Design review of the part built by this model. Coordinates are the model's own, in mm. A direction names the side the tool comes from. Coordinates: 2 decimals unless noted, no trailing zeros. Loops run counter-clockwise (first coordinate to the right, second up) from the corner with the lowest first, then second, coordinate; pieces in that order, holes last.
from build123d import *

# Parameters (mm, degrees)
SKETCH1_W           = 18.669
SKETCH1_H           = 50.8
BOSS_EXTRUDE1_DEPTH = 44.069
SKETCH2_W           = 44.069
SKETCH2_H           = 4.7625
CUT_EXTRUDE1_DEPTH  = 70.794328724
SKETCH3_W           = 44.069
SKETCH3_H           = 14.29004
CUT_EXTRUDE2_DEPTH  = 4.7625
SKETCH5_W           = 44.069
SKETCH5_H           = 14.29004
CUT_EXTRUDE3_DEPTH  = 4.7625
SKETCH4_W           = 18.669
SKETCH4_H           = 14.29004
CUT_EXTRUDE4_DEPTH  = 4.7625
SKETCH6_W           = 18.669
SKETCH6_H           = 14.29004
CUT_EXTRUDE5_DEPTH  = 4.7625
FILLET1_R           = 4.50088
FILLET2_R           = 2.49936
SKETCH7_R           = 2.5527
SKETCH7_R_2         = 2.54
CUT_EXTRUDE6_DEPTH  = 70.794328724
SKETCH8_R           = 2.0193
CUT_EXTRUDE7_DEPTH  = 69.673921566


with BuildPart() as part:
    # Sketch1 → Boss-Extrude1 (new body)
    with BuildSketch(Plane.XY):
        with Locations((9.3345, 25.4)):
            Rectangle(SKETCH1_W, SKETCH1_H)
    extrude(amount=BOSS_EXTRUDE1_DEPTH)

    # Sketch2 → Cut-Extrude1 (cut, through all)
    with BuildSketch(Plane(origin=(18.669, 0, 0), x_dir=(0, 0, -1), z_dir=(1, 0, 0))):
        with Locations((-22.0345, 2.38125)):
            Rectangle(SKETCH2_W, SKETCH2_H)
    extrude(amount=-CUT_EXTRUDE1_DEPTH, mode=Mode.SUBTRACT)

    # Sketch3 → Cut-Extrude2 (cut)
    with BuildSketch(Plane(origin=(18.669, 0, 0), x_dir=(0, 0, -1), z_dir=(1, 0, 0))):
        with Locations((-22.0345, 11.90752)):
            Rectangle(SKETCH3_W, SKETCH3_H)
    extrude(amount=-CUT_EXTRUDE2_DEPTH, mode=Mode.SUBTRACT)

    # Sketch5 → Cut-Extrude3 (cut)
    with BuildSketch(Plane.ZY):
        with Locations((22.0345, 11.90752)):
            Rectangle(SKETCH5_W, SKETCH5_H)
    extrude(amount=-CUT_EXTRUDE3_DEPTH, mode=Mode.SUBTRACT)

    # Sketch4 → Cut-Extrude4 (cut)
    with BuildSketch(Plane.XY.offset(44.069)):
        with Locations((9.3345, 11.90752)):
            Rectangle(SKETCH4_W, SKETCH4_H)
    extrude(amount=-CUT_EXTRUDE4_DEPTH, mode=Mode.SUBTRACT)

    # Sketch6 → Cut-Extrude5 (cut)
    with BuildSketch(Plane(origin=(0, 0, 0), x_dir=(-1, 0, 0), z_dir=(0, 0, -1))):
        with Locations((-9.3345, 11.90752)):
            Rectangle(SKETCH6_W, SKETCH6_H)
    extrude(amount=-CUT_EXTRUDE5_DEPTH, mode=Mode.SUBTRACT)

    # Fillet1
    fillet1_edges = [part.edges().sort_by_distance(p)[0] for p in [
        (4.7625, 11.90752, 39.3065),
        (13.9065, 11.90752, 39.3065),
        (4.7625, 11.90752, 4.7625),
        (13.9065, 11.90752, 4.7625),
    ]]
    fillet(fillet1_edges, radius=FILLET1_R)

    # Fillet2
    fillet2_edges = [part.edges().sort_by_distance(p)[0] for p in [
        (18.669, 34.92627, 0),
        (18.669, 34.92627, 44.069),
        (0, 34.92627, 44.069),
        (0, 34.92627, 0),
    ]]
    fillet(fillet2_edges, radius=FILLET2_R)

    # Sketch7 → Cut-Extrude6 (cut, through all)
    with BuildSketch(Plane.ZY):
        with Locations((9.52588, 38.1)):
            Circle(SKETCH7_R)
        with Locations((34.92588, 38.1)):
            Circle(SKETCH7_R_2)
        with Locations((34.92588, 25.4)):
            Circle(SKETCH7_R)
        with Locations((9.52588, 25.4)):
            Circle(SKETCH7_R)
    extrude(amount=-CUT_EXTRUDE6_DEPTH, mode=Mode.SUBTRACT)

    # Sketch8 → Cut-Extrude7 (cut, through all)
    with BuildSketch(Plane.ZY.offset(-4.7625)):
        with Locations((22.03538, 12.7)):
            Circle(SKETCH8_R)
        with Locations(Location((34.73538, 12.7, 0), (0, 0, 88.006602506))):
            Circle(SKETCH8_R)
        with Locations(Location((9.33538, 12.7, 0), (0, 0, 92.043366879))):
            Circle(SKETCH8_R)
    extrude(amount=-CUT_EXTRUDE7_DEPTH, mode=Mode.SUBTRACT)


solid = part.part
Q1. Take a section at D-D, the plane x = 17.25. Write out the cut boundary in (y, z), then the cut area to 3 significant figures.
Q2. Take a section at B-B, the plane x = 7. Write out the cut boundary in (y, z).
Q3. Take a section at A-A, the plane y = 38.1. Write out the cut boundary in (x, z), then the cut area to 3 significant figures.
Q4. The part is to be moulded in two halves that separate along Z. For faces 5 (the flat face through (4.762, 10, 22)), 6 (the cylindrical face through (9.204, 27.125, 7.644)), 7 (the flat face through (9, 35, 44.069)), say which applies: pulls with the +Z half, pulls with the -Z half, needs draft (parallel to the pull), parting line crosses it, or undercut.
Q5. Machinability: for faces 1 (the flat face through (3, 19.053, 22)), 2 (the cylindrical face through (6.046, 11.807, 6.116)), 3 (the cylindrical face through (12.553, 12.008, 6.046)), 4 (the cylindrical face through (12.553, 11.807, 38.023)), which of the approach directions +Z, -Z, +X, -X, +Y, -Y give a long, thin tool a straight path to every point of the face, cutting with its end or side? Answer none if there is none.
Q6. For line 1 (Y direction, x = 4, z = 35); line 2 (Z direction, x = 11.5, y = 36.5); line 3 (Y direction, x = 16, z = 7.5), list the stretches that pass through material, from the lowest coordinate up.
Q7. Clearance check with flat-ended pins moving along their axes: pin 1 Ø6 at (y, z) = (25.4, 9.53) entering from +X; pin 2 Ø4.5 at (y, z) = (12.7, 9.34) entering from -X; pin 3 Ø5 at (y, z) = (12.5, 10) entering from +X. State where each tip first meets the part, or that it passes through.
Q8. Take a section at C-C, the plane y = 11.5. Write out the cut boundary in (x, z).
Entries:
1. outline: (19.05, 0.25) - (50.8, 0.25) - (50.8, 43.82) - (19.05, 43.82) - close; hole circle Ø5.11 at (25.4, 9.53); hole circle Ø5.11 at (25.4, 34.93); hole circle Ø5.11 at (38.1, 9.53); hole circle Ø5.08 at (38.1, 34.93)
1. area: 1,300 mm2
2. outline: (4.76, 5.37) - (19.05, 5.37) - (19.05, 0) - (50.8, 0) - (50.8, 44.07) - (19.05, 44.07) - (19.05, 38.7) - (4.76, 38.7) - close; hole circle Ø4.04 at (12.7, 9.34); hole circle Ø4.04 at (12.7, 22.04); hole circle Ø4.04 at (12.7, 34.74); hole circle Ø5.11 at (25.4, 9.53); hole circle Ø5.11 at (25.4, 34.93); hole circle Ø5.11 at (38.1, 9.53); hole circle Ø5.08 at (38.1, 34.93)
3. outline: (0, 2.5) arc R2.5 ccw to (2.5, 0) - (16.17, 0) arc R2.5 ccw to (18.67, 2.5) - (18.67, 6.97) - (0, 6.97) - close; (0, 12.08) - (18.67, 12.08) - (18.67, 32.39) - (0, 32.39) - close; (0, 37.47) - (18.67, 37.47) - (18.67, 41.57) arc R2.5 ccw to (16.17, 44.07) - (2.5, 44.07) arc R2.5 ccw to (0, 41.57) - close
3. area: 627 mm2
4. face 5: needs draft
4. face 6: undercut
4. face 7: pulls with the +Z half
5. face 1: -Y
5. face 2: -Z, -X, -Y
5. face 3: -Z, +X, -Y
5. face 4: +Z, +X, -Y
6. line 1: y = 19.05 to 22.85, 27.95 to 35.56, 40.64 to 50.8
6. line 2: z = 0 to 7.54, 11.51 to 32.95, 36.9 to 44.07
6. line 3: y = 19.05 to 23.85, 26.95 to 36.55, 39.65 to 50.8
7. pin 1: stops at x = 18.67
7. pin 2: stops at x = 4.76
7. pin 3: stops at x = 13.91
8. outline: (4.76, 10.96) - (13.91, 10.96) - (13.91, 20.41) - (4.76, 20.41) - close; (4.76, 23.66) - (13.91, 23.66) - (13.91, 33.11) - (4.76, 33.11) - close; (5.04, 7.71) arc R4.5 ccw to (9.26, 4.76) - (9.41, 4.76) arc R4.5 ccw to (13.63, 7.71) - close; (5.04, 36.36) - (13.63, 36.36) arc R4.5 ccw to (9.41, 39.31) - (9.26, 39.31) arc R4.5 ccw to start
